Part print with two shaded views. Sizes in mm from the minimum x, y, z corner. A direction names the side the tool comes from. Round coordinates to 2 decimals unless told otherwise and drop trailing zeros. Loops run counter-clockwise (first coordinate to the right, second up) from the corner with the lowest first, then second, coordinate; pieces in that order, holes last. Notation, with made-up numbers: (15.25, 88) -> (47.25, 88) arc R30 ccw to (47.25, 116) -> close; hole circle Ø6 at (-13.5, -12). An arc over 180 degrees is marked (long way). Use a Markdown table: item, result. Add a question column.
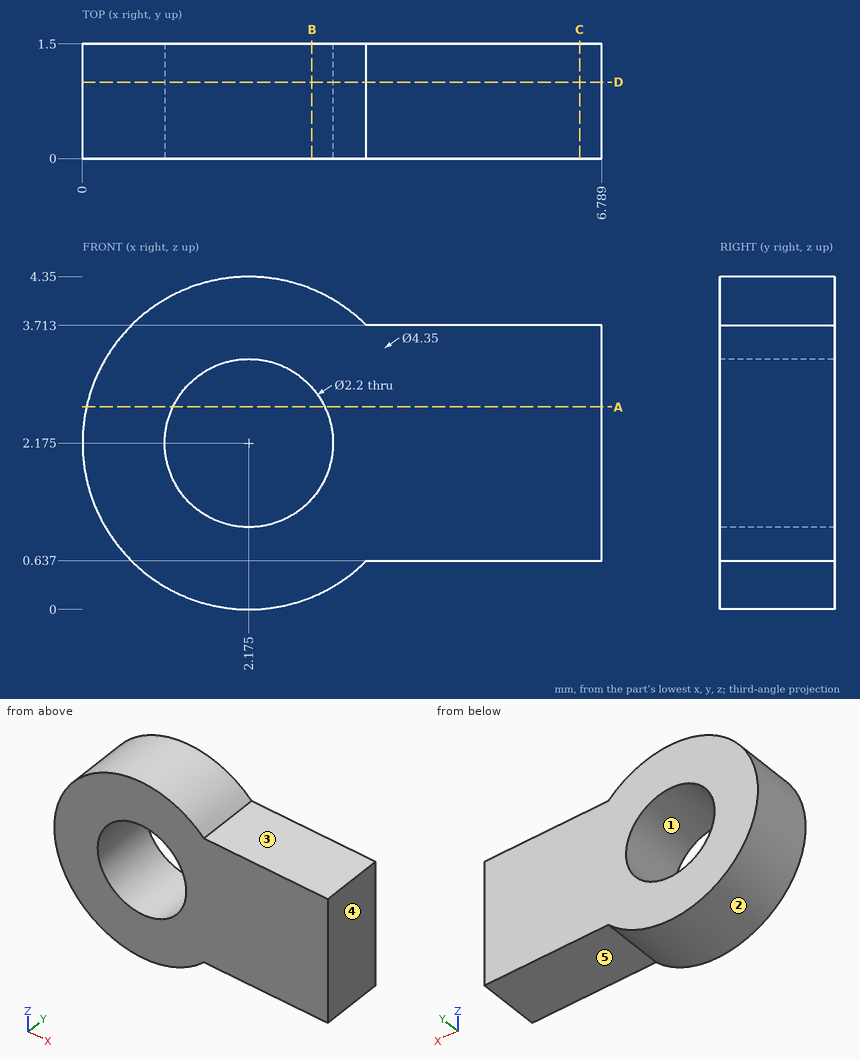
1) Cut at B-B on x = 3. Write the cut outline in (y, z).
2) Pull direction Z, two halves, no side cores. Call the marked faces 1, 2 and 3: +Z half, -Z half, draft (parallel to the pull), parting line (faces both ways), or undercut.
3) Wall check: probe 1 along Z at (x, y) = (2.75, 0.3); probe 2 along Z at (x, y) = (5, 1.45); probe 3 along X at (y, z) = (0.75, 2.5). Give the ranges that are in metal, low to high. Write a range as from..to.
4) Pin check, flat tips, straight feed: pin 1 Ø0.8 at (x, y) = (5, 1) entering from -Z; pin 2 Ø0.8 at (x, y) = (5.5, 0.5) entering from +Z. Stop position of each tip, or through.
5) Cut at A-A on z = 2.65. Write the cut outline in (x, y).
6) Cut at C-C on x = 6.5. Write the cut outline in (y, z).
7) Tool access for the marked faces 4 and 5: list every direction of +Z, -Z, +X, -X, +Y, -Y with a clear straight run to the whole face (end or side of a thin tool).
8) Cut at D-D on y = 1. Write the cut outline in (x, z) (3 decimals), and give its area (3 significant figures).
Established:
| question | item | result |
|---|---|---|
| 1 | outline | (0, 0.16) -> (1.5, 0.16) -> (1.5, 1.45) -> (0, 1.45) -> close; (0, 2.9) -> (1.5, 2.9) -> (1.5, 4.19) -> (0, 4.19) -> close |
| 2 | face 1 | undercut |
| 2 | face 2 | parting line |
| 2 | face 3 | +Z half |
| 3 | probe 1 | z = 0.08..1.24, 3.11..4.27 |
| 3 | probe 2 | z = 0.64..3.71 |
| 3 | probe 3 | x = 0.02..1.12, 3.23..6.79 |
| 4 | pin 1 | stops at z = 0.64 |
| 4 | pin 2 | stops at z = 3.71 |
| 5 | outline | (0.05, 0) -> (1.18, 0) -> (1.18, 1.5) -> (0.05, 1.5) -> close; (3.17, 0) -> (6.79, 0) -> (6.79, 1.5) -> (3.17, 1.5) -> close |
| 6 | outline | (0, 0.64) -> (1.5, 0.64) -> (1.5, 3.71) -> (0, 3.71) -> close |
| 7 | face 4 | +Z, -Z, +X, +Y, -Y |
| 7 | face 5 | -Z, +X, +Y, -Y |
| 8 | outline | (3.713, 0.637) -> (6.789, 0.637) -> (6.789, 3.713) -> (3.713, 3.713) arc R2.175 ccw (long way) to start; hole circle Ø2.2 at (2.175, 2.175) |
| 8 | area | 19.2 mm^2 |
